```python
from build123d import *

# Parameters (mm, degrees)
EXTRUDE_1_DEPTH          = 4
SKETCH_2_W               = 80
SKETCH_2_H               = 57
EXTRUDE_2_DEPTH          = 4
FILLET_1_R               = 2
SKETCH_3_R               = 2.1
CUT_EXTRUDE_1_DEPTH      = 61.340699366
SKETCH_4_R               = 2.1
EXTRUDE_3_DEPTH          = 5
SKETCH_5_W               = 46
SKETCH_5_H               = 2.95
EXTRUDE_4_DEPTH          = 12
CUT_EXTRUDE_2_DEPTH      = 89.843964342
CUT_EXTRUDE_2_DEPTH_BACK = 89.843964342
SKETCH_6_R               = 2.1
FILLET_2_R               = 3
SKETCH_7_W               = 7
SKETCH_7_H               = 1.5
CUT_EXTRUDE_3_DEPTH      = 15
MIRROR_3_COPY_1_SKETCH_W = 7
MIRROR_3_COPY_1_SKETCH_H = 1.5
MIRROR_3_COPY_1_DEPTH    = 15
CUT_EXTRUDE_4_DEPTH      = 10


with BuildPart() as part:
    # 草图1 → 凸台-拉伸1 (new body)
    with BuildSketch(Plane(origin=(0, 0, 0), x_dir=(1, 0, 0), z_dir=(0, 1, 0))):
        with BuildLine():
            Line((-20, -45), (20, -45))
            ThreePointArc((20, -45), (22.121320344, -44.121320344), (23, -42))
            Line((23, -42), (23, 42))
            ThreePointArc((23, 42), (22.121320344, 44.121320344), (20, 45))
            Line((20, 45), (-20, 45))
            ThreePointArc((-20, 45), (-22.121320344, 44.121320344), (-23, 42))
            Line((-23, 42), (-23, -42))
            ThreePointArc((-23, -42), (-22.121320344, -44.121320344), (-20, -45))
        make_face()
    extrude(amount=EXTRUDE_1_DEPTH)

    # 草图2 → 凸台-拉伸2 (add)
    with BuildSketch(Plane(origin=(0, 4, 0), x_dir=(1, 0, 0), z_dir=(0, 1, 0))):
        Rectangle(SKETCH_2_W, SKETCH_2_H)
    extrude(amount=-EXTRUDE_2_DEPTH)

    # 圆角1
    fillet_1_edges = [part.edges().sort_by_distance(p)[0] for p in [
        (40, 2, 28.5),
        (-40, 2, -28.5),
        (40, 2, -28.5),
        (23, 2, 28.5),
        (-23, 2, 28.5),
        (-40, 2, 28.5),
        (23, 2, -28.5),
        (-23, 2, -28.5),
    ]]
    fillet(fillet_1_edges, radius=FILLET_1_R)

    # 草图3 → 切除-拉伸1 (cut, through all)
    with BuildSketch(Plane(origin=(0, 4, 0), x_dir=(1, 0, 0), z_dir=(0, 1, 0))):
        with Locations(Location((15, -37.5, 0), (0, 0, 270))):
            Circle(SKETCH_3_R)
        with Locations(Location((-15, -37.5, 0), (0, 0, 270))):
            Circle(SKETCH_3_R)
        with Locations(Location((-15, 37.5, 0), (0, 0, 270))):
            Circle(SKETCH_3_R)
        with Locations(Location((15, 37.5, 0), (0, 0, 270))):
            Circle(SKETCH_3_R)
    extrude(amount=-CUT_EXTRUDE_1_DEPTH, mode=Mode.SUBTRACT)

    # 草图4 → 凸台-拉伸3 (add, symmetric)
    # profile 1 of 2: a face of its own
    with BuildSketch(Plane.XY):
        with BuildLine():
            ThreePointArc((-25.036748961, 16.605094313), (-30, 21), (-34.963251039, 16.605094313))
            Line((-34.963251039, 16.605094313), (-36.5, 4))
            Line((-36.5, 4), (-23.5, 4))
            Line((-23.5, 4), (-25.036748961, 16.605094313))
        make_face()
        with Locations((-30, 9)):
            Circle(SKETCH_4_R, mode=Mode.SUBTRACT)
        with Locations((-30, 16)):
            Circle(SKETCH_4_R, mode=Mode.SUBTRACT)
    # profile 2 of 2: a face of its own
    with BuildSketch(Plane.XY):
        with BuildLine():
            ThreePointArc((34.963251039, 16.605094313), (30, 21), (25.036748961, 16.605094313))
            Line((25.036748961, 16.605094313), (23.5, 4))
            Line((23.5, 4), (36.5, 4))
            Line((36.5, 4), (34.963251039, 16.605094313))
        make_face()
        with Locations((30, 9)):
            Circle(SKETCH_4_R, mode=Mode.SUBTRACT)
        with Locations((30, 16)):
            Circle(SKETCH_4_R, mode=Mode.SUBTRACT)
    extrude(amount=EXTRUDE_3_DEPTH, both=True)

    # 草图5 → 凸台-拉伸4 (add)
    with BuildSketch(Plane.XZ):
        Polygon((23, 31.5), (-23, 31.5), (-23, 30.5), (-23, 28.55), (23, 28.55), (23, 30.5), align=None)
        with Locations((0, 21.975)):
            Rectangle(SKETCH_5_W, SKETCH_5_H)
    extrude_4 = extrude(amount=EXTRUDE_4_DEPTH)

    # 镜向1: 凸台-拉伸4 across plane
    add(extrude_4.mirror(Plane.XY))

    # 草图6 → 切除-拉伸2 (cut, two sides: drawn at the far end of the back side and taken through both)
    with BuildSketch(Plane.XY.offset(31.5).offset(-CUT_EXTRUDE_2_DEPTH_BACK)):
        with Locations((19, -5.5)):
            Circle(SKETCH_6_R)
        with Locations((-19, -5.5)):
            Circle(SKETCH_6_R)
    extrude(amount=CUT_EXTRUDE_2_DEPTH + CUT_EXTRUDE_2_DEPTH_BACK, mode=Mode.SUBTRACT)

    # 圆角2
    fillet_2_edges = [part.edges().sort_by_distance(p)[0] for p in [
        (23, -12, 30.025),
        (-23, -12, 30.025),
        (23, -12, 21.975),
        (-23, -12, 21.975),
        (-23, -12, -30.025),
        (23, -12, -30.025),
        (-23, -12, -21.975),
        (23, -12, -21.975),
    ]]
    fillet(fillet_2_edges, radius=FILLET_2_R)

    # 草图7 → 切除-拉伸3 (cut)
    with BuildSketch(Plane.ZY.offset(40)):
        with Locations((-20, 0.75)):
            Rectangle(SKETCH_7_W, SKETCH_7_H)
    cut_extrude_3 = extrude(amount=-CUT_EXTRUDE_3_DEPTH, mode=Mode.SUBTRACT)

    # 镜向2: 切除-拉伸3 across plane
    add(cut_extrude_3.mirror(Plane.XY), mode=Mode.SUBTRACT)

    # 镜向3: 切除-拉伸3 across plane
    add(cut_extrude_3.mirror(Plane(origin=(0, 0, 0), x_dir=(0, 0, 1), z_dir=(1, 0, 0))), mode=Mode.SUBTRACT)

    # 镜向3 copy 1 sketch → 镜向3 copy 1 (cut)
    with BuildSketch(Plane(origin=(40, 0, 0), x_dir=(0, 0, -1), z_dir=(1, 0, 0))):
        with Locations((-20, 0.75)):
            Rectangle(MIRROR_3_COPY_1_SKETCH_W, MIRROR_3_COPY_1_SKETCH_H)
    extrude(amount=-MIRROR_3_COPY_1_DEPTH, mode=Mode.SUBTRACT)

    # 草图8 → 切除-拉伸4 (cut)
    with BuildSketch(Plane(origin=(0, 4, 0), x_dir=(1, 0, 0), z_dir=(0, 1, 0))):
        with BuildLine():
            Line((-5, -16), (5, -16))
            ThreePointArc((5, -16), (7.121320344, -15.121320344), (8, -13))
            Line((8, -13), (8, 13))
            ThreePointArc((8, 13), (7.121320344, 15.121320344), (5, 16))
            Line((5, 16), (-5, 16))
            ThreePointArc((-5, 16), (-7.121320344, 15.121320344), (-8, 13))
            Line((-8, 13), (-8, -13))
            ThreePointArc((-8, -13), (-7.121320344, -15.121320344), (-5, -16))
        make_face()
    extrude(amount=-CUT_EXTRUDE_4_DEPTH, mode=Mode.SUBTRACT)


solid = part.part
```
Read the model definition and answer for the solid it produces. Units are mm, in the model's axes. A direction names the side the tool comes from. Give positions to 0.01 mm unless a question says otherwise; leave off trailing zeros. Loops run counter-clockwise (first coordinate to the right, second up) from the corner with the lowest first, then second, coordinate; pieces in that order, holes last.
Item 1: The part is cut by section D-D (x = -19). Give the number of separate pieces and of enclosed holes in the cut face, and give its area (3 significant figures).
Item 2: For faces 4 (the flat face through (-23, -4, -22)), 5 (the flat face through (0, -6, -23.45)), 6 (the flat face through (-23, 0.5, -33.9)), 7 (the cylindrical face through (7.14, 2.03, -15.1)), determine the directions among +Z, -Z, +X, -X, +Y, -Y from which every point of the face is accessible in a straight line to the end or side of a thin tool.
Item 3: Each of these flat-tipped pins is pushed along its axis until it touches: pin 1 Ø0.9 at (y, z) = (-2.5, -21.5) entering from +X; pin 2 Ø3.5 at (x, z) = (32.5, 19.5) entering from -Y; pin 3 Ø6.5 at (x, z) = (15, -37.5) entering from -Y. Where does it stop, or does it pass through?
Item 4: Find the intervals of material crossed by line 1 along Y through (x, z) = (30, -1); line 2 along Z through (x, y) = (18, -9); line 3 along X through (y, z) = (1.9, -37.5), in increasing order.
Item 5: The part is cut by section C-C (z = 37.5). Write down the section's boundary in (x, y).
Item 6: The part is cut by section A-A (z = 12). Write down the section's boundary in (x, y), and give its area (3 significant figures).
Item 7: The part is cut by section B-B (x = -30). Write down the section's boundary in (y, z).
Item 8: The mould has two halves that part along X. Classify faces 1 (the flat face through (-23, -4, 22)), 2 (the cylindrical face through (39.4, 1.97, -27.93)), 3 (the cylindrical face through (-30, 21, 0)): released by +X, released by -X, zero draft, split by the parting line, or undercut.
Taken from the geometry:
1. separate pieces: 5
1. enclosed holes: 0
1. area: 452 mm2
2. face 4: +Z, -Z, -X, -Y
2. face 5: +X, -X, -Y
2. face 6: -Z, -X, -Y
2. face 7: +Y, -Y
3. pin 1: stops at x = 23
3. pin 2: stops at y = 1.5
3. pin 3: stops at y = 0
4. line 1: y = 0 to 6.9, 11.1 to 13.9, 18.1 to 21
4. line 2: z = -31.5 to -28.55, -23.45 to -20.5, 20.5 to 23.45, 28.55 to 31.5
4. line 3: x = -23 to -17.1, -12.9 to 12.9, 17.1 to 23
5. outline: (-23, 0) - (-17.1, 0) - (-17.1, 4) - (-23, 4) - close; (-12.9, 0) - (12.9, 0) - (12.9, 4) - (-12.9, 4) - close; (17.1, 0) - (23, 0) - (23, 4) - (17.1, 4) - close
6. outline: (-40, 0) - (-8, 0) - (-8, 4) - (-40, 4) - close; (8, 0) - (40, 0) - (40, 4) - (8, 4) - close
6. area: 256 mm2
7. outline: (0, -28.5) - (4, -28.5) - (4, -5) - (6.9, -5) - (6.9, 5) - (4, 5) - (4, 28.5) - (0, 28.5) - (0, 23.5) - (1.5, 23.5) - (1.5, 16.5) - (0, 16.5) - (0, -16.5) - (1.5, -16.5) - (1.5, -23.5) - (0, -23.5) - close; (11.1, -5) - (13.9, -5) - (13.9, 5) - (11.1, 5) - close; (18.1, -5) - (21, -5) - (21, 5) - (18.1, 5) - close
8. face 1: released by -X
8. face 2: released by +X
8. face 3: undercut
